Geometry check sheet. Reference: drawing and pictorial views, mm from the part's lowest x, y, z. A direction names the side the tool comes from. Give positions to 0.01 mm unless a question says otherwise; leave off trailing zeros. Write each loop counter-clockwise with the first axis right and the second up, starting at its lowest first coordinate (ties: lowest second). Pieces come first, ordered by that corner, then holes. Notation, with made-up numbers: M 77.25,67.5 L 87.25,67.5 A19 cw 87.25,93.5 Z; hole C 71.5,-13 d7. An arc over 180 degrees is marked long. Answer as a JSON object with one key per item and string values.
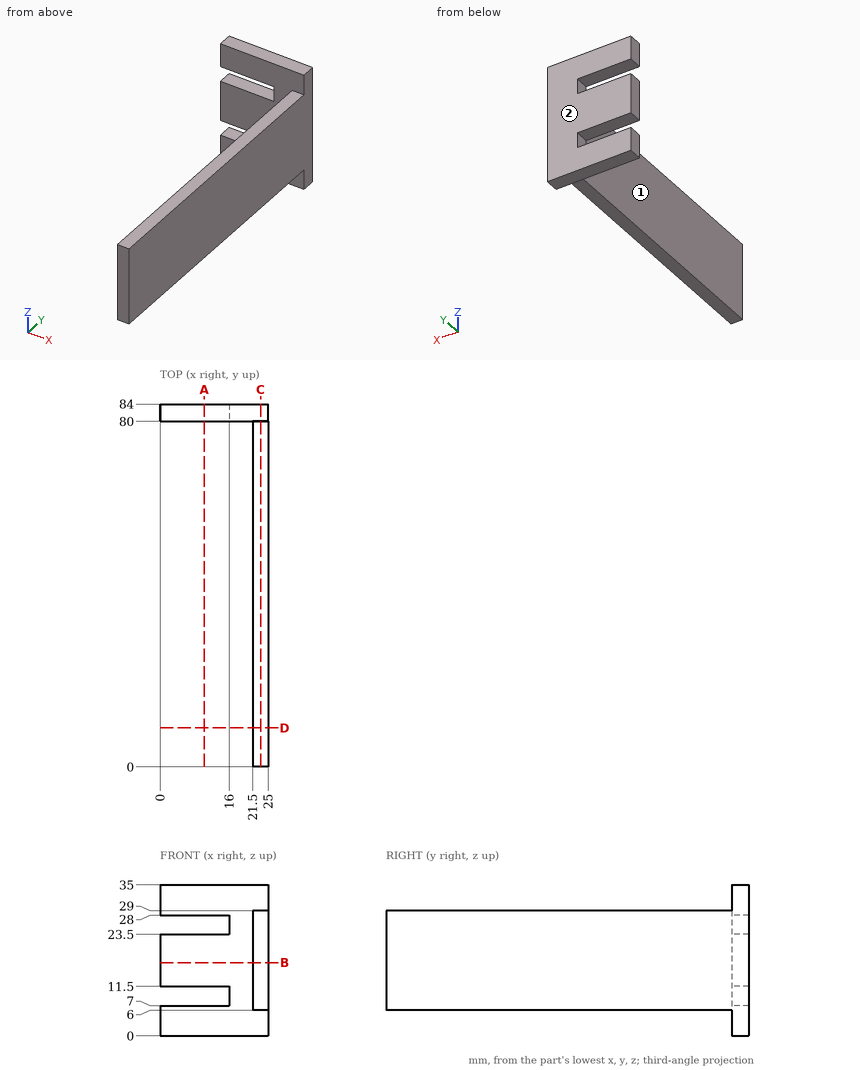
1) Access from +Z, -Z, +X, -X, +Y, -Y to the whole of each face (thin tool, end or side, straight path). Record for the marked faces 1 and 2.
Completed:
{"face 1": "+Z, -Z, -X, -Y", "face 2": "+Z, -Z, +X, -X, +Y"}
2) Section check D-D on y = 9. Record the boundary of the cut face in (x, z), and give its area (3 significant figures).
Completed:
{"outline": "M 21.5,6 L 25,6 L 25,29 L 21.5,29 Z", "area": "80.5 mm2"}
3) Section check C-C on x = 23.25. Record the boundary of the cut face in (y, z).
Completed:
{"outline": "M 0,6 L 80,6 L 80,0 L 84,0 L 84,35 L 80,35 L 80,29 L 0,29 Z"}
4) Thickness scan on L1, parallel to X at y = 48.5, z = 10; L2, parallel to Y at x = 3.75, z = 14; L3, parallel to Z at x = 23, y = 77.5. Record the ranges inside material, lowest first.
Completed:
{"L1": "x = 21.5 to 25", "L2": "y = 80 to 84", "L3": "z = 6 to 29"}
5) Section check B-B on z = 17. Record the boundary of the cut face in (x, y).
Completed:
{"outline": "M 0,80 L 21.5,80 L 21.5,0 L 25,0 L 25,84 L 0,84 Z"}
6) Section check A-A on x = 10.25. Record the boundary of the cut face in (y, z), and give its area (3 significant figures).
Completed:
{"outline": "M 80,0 L 84,0 L 84,7 L 80,7 Z; M 80,11.5 L 84,11.5 L 84,23.5 L 80,23.5 Z; M 80,28 L 84,28 L 84,35 L 80,35 Z", "area": "104 mm2"}
7) Go/stop test with flat-tipped pins: pin 1 (3 mm diameter, centred on x = 23, y = 51.5, fed in from -Z); pin 2 (3 mm diameter, centred on x = 23, y = 41.5, fed in from +Z); pin 3 (4.5 mm diameter, centred on y = 82.5, z = 8.5, fed in from -X); pin 4 (6 mm diameter, centred on x = 11.5, z = 15, fed in from -Y). Record where each tip stops, or that it passes through.
Completed:
{"pin 1": "stops at z = 6", "pin 2": "stops at z = 29", "pin 3": "stops at x = 0", "pin 4": "stops at y = 80"}
